from build123d import *

# Parameters (mm, degrees)
F0_W     = 1346.2
F0_H     = 685.8
F1_DEPTH = 25.4
F2_W     = 50.8
F2_H     = 317.5
F3_DEPTH = 38.1
F4_W     = 50.8
F4_H     = 76.2
F5_DEPTH = 660.4
F7_DEPTH = 25.4
F8_W     = 1193.8
F8_H     = 50.8
F9_DEPTH = 304.8


with BuildPart() as f1:
    # F0 (on Front) → F1 (new body)
    with BuildSketch(Plane.XZ):
        with Locations((-279.338504, 78.177206)):
            Rectangle(F0_W, F0_H)
    extrude(amount=F1_DEPTH)

    # F2 (on face) → F3 (join)
    with BuildSketch(Plane.XZ.offset(25.4)):
        with Locations((-905.169547, 132.599801)):
            Rectangle(F2_W, F2_H)
        with Locations((346.49254, 132.599801)):
            Rectangle(F2_W, F2_H)
    extrude(amount=F3_DEPTH)

    # F4 (on face) → F5 (join)
    with BuildSketch(Plane.XZ.offset(25.4)):
        with Locations((-905.597014, -66.111187)):
            Rectangle(F4_W, F4_H)
        with Locations((346.920007, -66.111187)):
            Rectangle(F4_W, F4_H)
    extrude(amount=F5_DEPTH)

    # F6 (on face) → F7 (join)
    with BuildSketch(Plane.XZ.offset(685.8)):
        with BuildLine():
            Line((-880.196954, -138.340718), (-880.196954, 318.859282))
            ThreePointArc((-880.196954, 318.859282), (-887.636442, 336.819794), (-905.596954, 344.259282))
            ThreePointArc((-905.596954, 344.259282), (-923.557467, 336.819794), (-930.996954, 318.859282))
            Line((-930.996954, 318.859282), (-930.996954, -138.340718))
            ThreePointArc((-930.996954, -138.340718), (-923.557467, -156.30123), (-905.596954, -163.740718))
            ThreePointArc((-905.596954, -163.740718), (-887.636442, -156.30123), (-880.196954, -138.340718))
        make_face()
        with BuildLine():
            ThreePointArc((346.919947, 344.259282), (328.959435, 336.819794), (321.519947, 318.859282))
            Line((321.519947, 318.859282), (321.519947, -138.340718))
            ThreePointArc((321.519947, -138.340718), (328.959435, -156.30123), (346.919947, -163.740718))
            ThreePointArc((346.919947, -163.740718), (364.88046, -156.30123), (372.319947, -138.340718))
            Line((372.319947, -138.340718), (372.319947, 318.859282))
            ThreePointArc((372.319947, 318.859282), (364.88046, 336.819794), (346.919947, 344.259282))
        make_face()
    extrude(amount=F7_DEPTH)

    # F8 (on face) → F9 (join)
    with BuildSketch(Plane.XZ.offset(25.4)):
        with Locations((-279.633806, -75.797988)):
            Rectangle(F8_W, F8_H)
    extrude(amount=F9_DEPTH)


solid = f1.part
Can you work these out from the model? Positions are in its coordinate system, mm. A direction names the side the tool comes from. Give positions to 0.01 mm unless a question says otherwise; leave off trailing zeros. Order: outer loops, then holes, each group sorted by start corner. A loop starts at its lowest first (then second) coordinate and runs counter-clockwise, first axis right, second up. Notation, with made-up numbers: M -21.75,57 L 34.25,57 A12 cw 34.25,70 Z; hole C 81.5,15 d8. An arc over 180 degrees is marked long. Use one line per item in the form item = value. Start each with the question number.
Item 1: If we section it at A-A (y = -312): Write out the boundary of the cut face in (x, z).
Item 2: If we section it at C-C (y = -399): Write out the boundary of the cut face in (x, z), then the cut area to 3 significant figures.
Item 3: For faces 4 (the flat face through (372.32, -351, -67)), 5 (the flat face through (-906, -685.8, 94)), 6 (the flat face through (346, -63.5, 135)), which set-ups out of +Z, -Z, +X, -X, +Y, -Y let a thin tool reach every point of the face, with its end or its side?
Item 4: We'd pull the mould along Y, two halves only. Please class faces 1 (the flat face through (347, -351, -104.211)), 2 (the flat face through (347, -711.2, 94)), 3 (the flat face through (372.32, -698, 87)): +Y half, -Y half, draft (parallel to the pull), parting line (faces both ways), or undercut.
Item 5: If we section it at D-D (x = -852): Write out the boundary of the cut face in (y, z).
Item 6: If I drill on line 1 along X through (y, z) = (-159.5, -65.5); line 2 along Y through (x, z) = (73.5, -194.5); line 3 along Z through (x, y) = (-279, -238), over which ranges is the centre line in solid material (lowest first)?
Item 7: If we section it at B-B (z = 58.5): Write out the boundary of the cut face in (x, y).
Item 8: Will these pins go through, and if not, where does the flat tip stop? pin 1 Ø15 at (x, z) = (-235, -66) entering from -Y; pin 2 Ø19 at (x, y) = (-898.5, -48) entering from +Z; pin 3 Ø10 at (x, z) = (-607.5, 59) entering from +Y; pin 4 Ø12.5 at (y, z) = (-696, 79) entering from -X.
Outcome:
q1.outline = M -931,-104.21 L -880.2,-104.21 L -880.2,-28.01 L -931,-28.01 Z; M -876.53,-101.2 L 317.27,-101.2 L 317.27,-50.4 L -876.53,-50.4 Z; M 321.52,-104.21 L 372.32,-104.21 L 372.32,-28.01 L 321.52,-28.01 Z
q2.outline = M -931,-104.21 L -880.2,-104.21 L -880.2,-28.01 L -931,-28.01 Z; M 321.52,-104.21 L 372.32,-104.21 L 372.32,-28.01 L 321.52,-28.01 Z
q2.area = 7,740 mm2
q3.face_4 = +Z, -Z, +X, -Y
q3.face_5 = +Z, +X, -X
q3.face_6 = +Z, +X, -X
q4.face_1 = undercut
q4.face_2 = -Y half
q4.face_3 = draft
q5.outline = M -330.2,-101.2 L -25.4,-101.2 L -25.4,-264.72 L 0,-264.72 L 0,421.08 L -25.4,421.08 L -25.4,-50.4 L -330.2,-50.4 Z
q6.line_1 = -931 to -880.2, -876.53 to 317.27, 321.52 to 372.32
q6.line_2 = -25.4 to 0
q6.line_3 = -101.2 to -50.4
q7.outline = M -952.44,-25.4 L -930.57,-25.4 L -930.57,-63.5 L -879.77,-63.5 L -879.77,-25.4 L 321.09,-25.4 L 321.09,-63.5 L 371.89,-63.5 L 371.89,-25.4 L 393.76,-25.4 L 393.76,0 L -952.44,0 Z; M -931,-711.2 L -880.2,-711.2 L -880.2,-685.8 L -931,-685.8 Z; M 321.52,-711.2 L 372.32,-711.2 L 372.32,-685.8 L 321.52,-685.8 Z
q8.pin_1 = -330.2
q8.pin_2 = 291.35
q8.pin_3 = 0
q8.pin_4 = -931
